from build123d import *

# Parameters (mm, degrees)
CROQUIS1_R              = 1.6
SALIENTE_EXTRUIR1_DEPTH = 10
CORTAR_EXTRUIR1_DEPTH   = 5.5
CORTAR_EXTRUIR2_REACH   = 12.696
CROQUIS3_R              = 1.6
CORTAR_EXTRUIR3_DEPTH   = 2.5


with BuildPart() as part:
    # Croquis1 → Saliente-Extruir1 (new body)
    with BuildSketch(Plane.XY):
        Polygon((17.180905327, 0), (5.936351089, 0), (0, 4.722097457), (0, 13.666629237), align=None)
        with Locations((7.975771065, 2.85)):
            Circle(CROQUIS1_R, mode=Mode.SUBTRACT)
    extrude(amount=SALIENTE_EXTRUIR1_DEPTH)

    # Croquis2 → Cortar-Extruir1 (cut)
    with BuildSketch(Plane.XY.offset(10)):
        Polygon((6.330322798, 0), (9.621219332, 0), (11.2666676, 2.85), (9.621219332, 5.7), (6.330322798, 5.7), (4.684874531, 2.85), align=None)
    extrude(amount=-CORTAR_EXTRUIR1_DEPTH, mode=Mode.SUBTRACT)

    # Croquis3 → Cortar-Extruir2 (cut, up to next)
    with BuildSketch(Plane(origin=(6.658212283, 8.370324012, 0), x_dir=(0.782601054, -0.622523566, 0), z_dir=(0.622523566, 0.782601054, 0)), mode=Mode.PRIVATE) as cortar_extruir2_sk1:
        with Locations((-1.507798766, -5)):
            Circle(CROQUIS3_R)
    cortar_extruir2_tool1 = extrude(cortar_extruir2_sk1.sketch, amount=-CORTAR_EXTRUIR2_REACH, mode=Mode.PRIVATE) & part.part
    add(cortar_extruir2_tool1.solids().sort_by_distance((5.478207, 9.308964, 5))[0], mode=Mode.SUBTRACT)

    # Croquis4 → Cortar-Extruir3 (cut)
    with BuildSketch(Plane(origin=(2.300547322, 2.892116633, 0), x_dir=(0.782601054, -0.622523566, 0), z_dir=(-0.622523566, -0.782601054, 0))):
        Polygon((1.783097769, 5), (0.137649502, 7.85), (-3.153247033, 7.85), (-4.7986953, 5), (-3.153247033, 2.15), (0.137649502, 2.15), align=None)
    extrude(amount=-CORTAR_EXTRUIR3_DEPTH, mode=Mode.SUBTRACT)


solid = part.part
Check sheet for the modelled part. Datum: model origin and axes. Units: mm. A direction names the side the tool comes from. Coordinates: 2 decimals unless noted, no trailing zeros. Write each loop counter-clockwise with the first axis right and the second up, starting at its lowest first coordinate (ties: lowest second). Pieces come first, ordered by that corner, then holes.
Item 1: Cross-section at D-D on y = 1. Record the boundary of the cut face in (x, z), then the cut area to 3 significant figures.
Numbers:
outline: (4.68, 0) - (15.92, 0) - (15.92, 10) - (10.2, 10) - (10.2, 4.5) - (5.75, 4.5) - (5.75, 10) - (4.68, 10) - close
area: 88.0 mm2
Item 2: Access from +Z, -Z, +X, -X, +Y, -Y to the whole of each face (thin tool, end or side, straight path). Record for faces 1 (the face through (3.828, 3.252, 6.405)), 2 (the face through (8, 5.7, 7)), 3 (the face through (5.5, 1.44, 7.29)).
Numbers:
face 1: -X
face 2: +Z, -Y
face 3: +Z
Item 3: Mould release check, pull along Z, two halves, no side actions. Record for faces 4 (the face through (0.48, 6.72, 3.28)), 5 (the face through (0.347, 6.511, 6.762)), 6 (the face through (10.455, 4.255, 7.288)), 7 (the face through (5, 5, 0)): released by +Z, released by -Z, zero draft, split by the parting line, or undercut.
Numbers:
face 4: undercut
face 5: undercut
face 6: zero draft
face 7: released by -Z
Item 4: Cross-section at A-A on x = 7.25. Record the boundary of the cut face in (y, z), then the cut area to 3 significant figures.
Numbers:
outline: (0, 0) - (1.42, 0) - (1.42, 4.5) - (0, 4.5) - close; (4.28, 0) - (7.9, 0) - (7.9, 10) - (5.7, 10) - (5.7, 4.5) - (4.28, 4.5) - close
area: 34.8 mm2
Item 5: Scan lines: probe 1 along Z at (x, y) = (5.25, 9); probe 2 along X at (y, z) = (8, 5.5); probe 3 along X at (y, z) = (11.75, 8.5). Record each from-to range of solid material in increasing order.
Numbers:
probe 1: z = 0 to 3.4, 6.6 to 10
probe 2: x = 0 to 2.49, 6.38 to 7.12
probe 3: x = 0 to 2.41
Item 6: Cross-section at C-C on z = 9.25. Record the boundary of the cut face in (x, y).
Numbers:
outline: (0, 4.72) - (5.94, 0) - (6.33, 0) - (4.68, 2.85) - (6.33, 5.7) - (9.62, 5.7) - (11.27, 2.85) - (9.62, 0) - (17.18, 0) - (0, 13.67) - close
Item 7: Depth check by flat-ended pin: pin 1 Ø3 at (y, z) = (8, 8.5) entering from +X; pin 2 Ø1.6 at (x, z) = (8, 7.5) entering from -Y; pin 3 Ø1.9 at (x, y) = (7.98, 2.85) entering from -Z; pin 4 Ø4 at (x, z) = (10.5, 9) entering from +Y. Enter the tip coordinate at first touch or a pass-through.
Numbers:
pin 1: stops at x = 9.01
pin 2: stops at y = 5.7
pin 3: passes through
pin 4: stops at y = 6.91
Item 8: Cross-section at B-B on z = 6. Record the boundary of the cut face in (x, y).
Numbers:
outline: (0, 6.78) - (0.55, 7.48) - (1.7, 6.56) - (4.5, 10.09) - (0, 13.67) - close; (3.24, 2.14) - (5.94, 0) - (6.33, 0) - (4.68, 2.85) - (6.33, 5.7) - (9.62, 5.7) - (11.27, 2.85) - (9.62, 0) - (17.18, 0) - (6.46, 8.53) - (3.65, 5.01) - (4.8, 4.1) - close
